Could you check a few things on this drawing? It's one solid part, dimensions in mm from its lowest x, y, z. Give positions to 0.01 mm unless a question says otherwise; leave off trailing zeros. Loops run counter-clockwise (first coordinate to the right, second up) from the corner with the lowest first, then second, coordinate; pieces in that order, holes last. Notation, with made-up numbers: M 75,29.5 L 93,29.5 A19 cw 93,61.5 Z; hole C 12,-35 d11. An arc over 180 degrees is marked long. Answer as a JSON object with one key per item and string values.
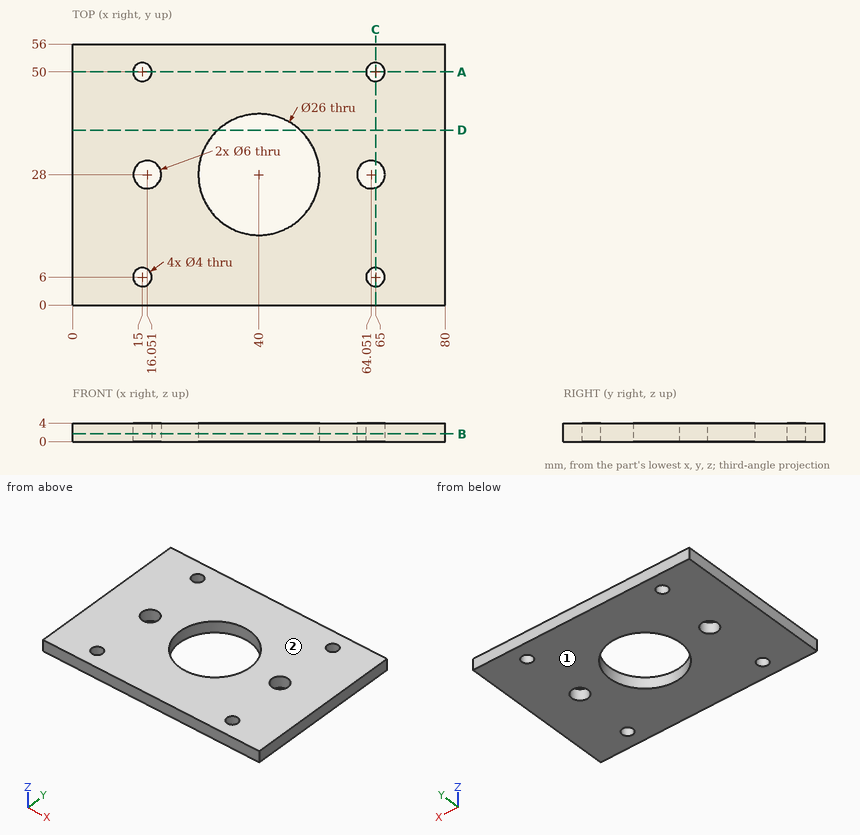
1) If we mould it in two halves opening along Z, with no side actions, what happens to the marked faces 1 and 2? For each: +Z half, -Z half, draft (parallel to the pull), parting line (faces both ways), or undercut.
Answer list:
{"face 1": "-Z half", "face 2": "+Z half"}
2) Suppose I cut it at C-C, the plane x = 65. Write out the boundary of the cut face in (y, z).
Answer list:
{"outline": "M 0,0 L 4,0 L 4,4 L 0,4 Z; M 8,0 L 25.15,0 L 25.15,4 L 8,4 Z; M 30.85,0 L 48,0 L 48,4 L 30.85,4 Z; M 52,0 L 56,0 L 56,4 L 52,4 Z"}
3) Suppose I cut it at D-D, the plane y = 37.5. Write out the boundary of the cut face in (x, z).
Answer list:
{"outline": "M 0,0 L 31.13,0 L 31.13,4 L 0,4 Z; M 48.87,0 L 80,0 L 80,4 L 48.87,4 Z"}
4) Please list where these lines run through material, in increasing order: line 1 along X through (y, z) = (5, 1.05); line 2 along Y through (x, z) = (65, 1.95); line 3 along X through (y, z) = (26.5, 3.65). Write a range as from..to.
Answer list:
{"line 1": "0..13.27, 16.73..63.27, 66.73..80", "line 2": "0..4, 8..25.15, 30.85..48, 52..56", "line 3": "0..13.45, 18.65..27.09, 52.91..61.45, 66.65..80"}
5) Suppose I cut it at B-B, the plane z = 1.7. Write out the boundary of the cut face in (x, y).
Answer list:
{"outline": "M 0,0 L 80,0 L 80,56 L 0,56 Z; hole C 15,6 d4; hole C 15,50 d4; hole C 16.05,28 d6; hole C 40,28 d26; hole C 64.05,28 d6; hole C 65,6 d4; hole C 65,50 d4"}
6) Suppose I cut it at A-A, the plane y = 50. Write out the boundary of the cut face in (x, z), and give its area (3 significant figures).
Answer list:
{"outline": "M 0,0 L 13,0 L 13,4 L 0,4 Z; M 17,0 L 63,0 L 63,4 L 17,4 Z; M 67,0 L 80,0 L 80,4 L 67,4 Z", "area": "288 mm^2"}
